Job drawing, mm, ordinate dimensions from the low corner. One solid piece. A direction names the side the tool comes from. Coordinates: 2 decimals unless noted, no trailing zeros. Write each loop counter-clockwise with the first axis right and the second up, starting at its lowest first coordinate (ties: lowest second). Pieces come first, ordered by that corner, then holes. Notation, with made-up numbers: (70, -32) - (95, -32) arc R29 ccw to (95, -8) - close; hole circle Ø5 at (-26, -27.5). An arc over 180 degrees is marked (long way). Put each result on its own line as item: value. Start each with the question number.
1. Saw through at C-C, the plane z = 63. Write the cut outline in (x, y) (1 decimal), plus the area to 3 significant figures.
2. Saw through at A-A, the plane x = 67. Write the cut outline in (y, z).
3. Drop flat-ended pins along their axis: P1, Ø12, axis at x = 59, y = 15, coming from the -Z side; P2, Ø2, axis at x = 37.5, y = 26.5, coming from the -Z side; P3, Ø8, axis at x = 16.5, y = 21, coming from the -Z side; P4, Ø3, axis at x = 70.5, y = 10.5, coming from the -Z side (1 decimal). Give the stop position or say it passes through.
4. Drill centre lines: L1, parallel to Z at x = 35, y = 10.5; L2, parallel to Y at x = 6.5, z = 23; L3, parallel to Z at x = 4, y = 5.5 (1 decimal). Where is each one in solid material? Low to high. Write a range as from..to.
5. Saw through at D-D, the plane z = 19. Write the cut outline in (x, y).
6. Which spindle directions (+Z, -Z, +X, -X, +Y, -Y) get a long thin tool onto all of the face, cutting with end or side? Do the marked faces 1, 2 and 3. Say none if no direction does.
7. Saw through at B-B, the plane y = 20. Write the cut outline in (x, z) (1 decimal), plus the area to 3 significant figures.
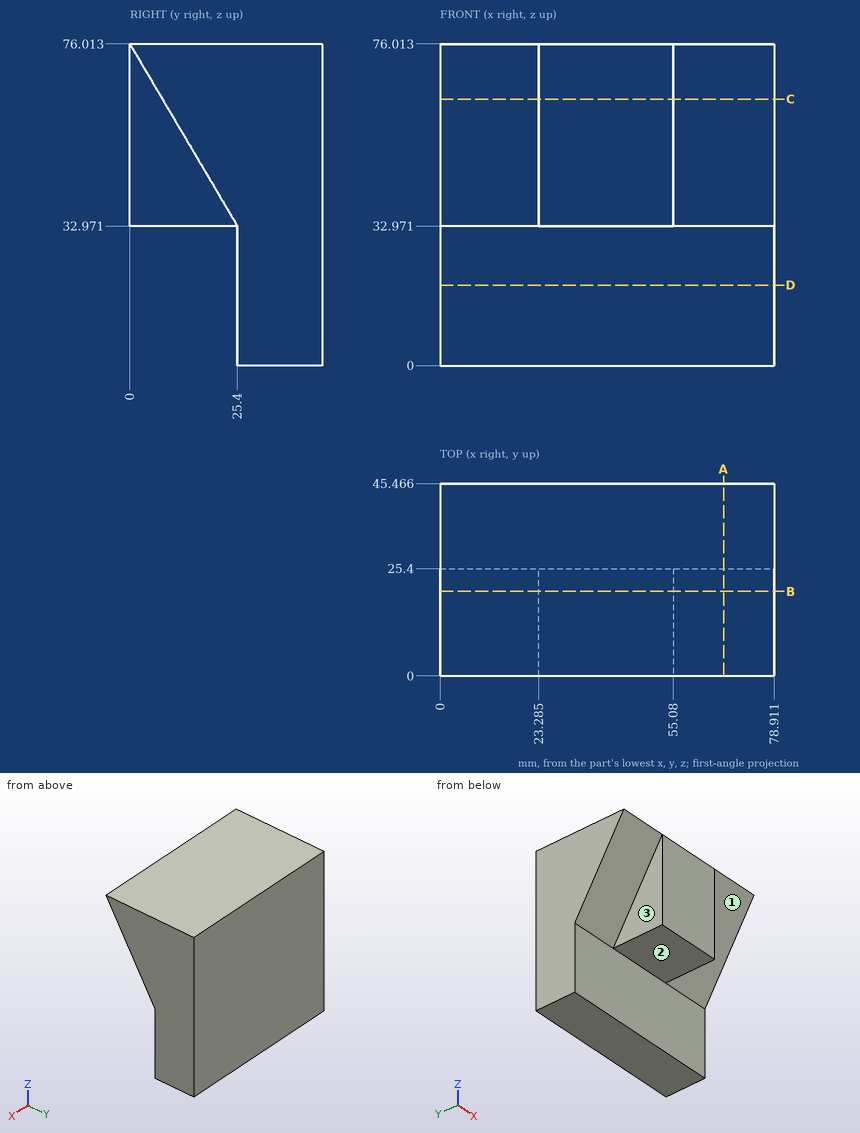
Final values:
1. outline: (0, 7.7) - (23.3, 7.7) - (23.3, 0) - (55.1, 0) - (55.1, 7.7) - (78.9, 7.7) - (78.9, 45.5) - (0, 45.5) - close
1. area: 3,230 mm²
2. outline: (0, 76.01) - (25.4, 32.97) - (25.4, 0) - (45.47, 0) - (45.47, 76.01) - close
3. P1: stops at z = 32.97
3. P2: stops at z = 0
3. P3: stops at z = 33.65
3. P4: stops at z = 55.7
4. L1: z = 32.97..76.01
4. L2: y = 25.4..45.47
4. L3: z = 66.7..76
5. outline: (0, 25.4) - (78.91, 25.4) - (78.91, 45.47) - (0, 45.47) - close
6. face 1: -Z, +X, -Y
6. face 2: -Z, +X, -X, -Y
6. face 3: -Z, -X, -Y
7. outline: (0, 42.1) - (23.3, 42.1) - (23.3, 33) - (55.1, 33) - (55.1, 42.1) - (78.9, 42.1) - (78.9, 76) - (0, 76) - close
7. area: 2,970 mm²
